Read the model definition and answer for the solid it produces. Units are mm, in the model's axes. Give positions to 0.01 mm unless a question says otherwise; leave off trailing zeros. Write each loop counter-clockwise with the first axis right and the second up, starting at its lowest first coordinate (ties: lowest second). Pieces come first, ordered by that corner, then holes. Notation, with made-up numbers: (60.5, -13.5) -> (102.5, -13.5) arc R12 cw to (102.5, -7.5) -> close; hole circle Ø5 at (-16.75, 33). An arc over 180 degrees is marked (long way). Use a Markdown table: item, result.
from build123d import *

# Parameters (mm, degrees)
BOSS_EXTRUDE1_DEPTH = 2
FILLET1_R           = 3


with BuildPart() as part:
    # Sketch1 → Boss-Extrude1 (new body)
    with BuildSketch(Plane(origin=(0, 0, 0), x_dir=(1, 0, 0), z_dir=(0, 1, 0))):
        Polygon((-160, -197.649746193), (-160, -185.649746193), (0, -185.649746193), (0, -197.649746193), (30, -197.649746193), (30, 34.350253807), (-190, 34.350253807), (-190, -197.649746193), align=None)
    extrude(amount=BOSS_EXTRUDE1_DEPTH)

    # Fillet1
    fillet1_edges = [part.edges().sort_by_distance(p)[0] for p in [
        (-190, 1, -34.350253807),
        (30, 1, -34.350253807),
        (30, 1, 197.649746193),
        (0, 1, 197.649746193),
        (-160, 1, 197.649746193),
        (-190, 1, 197.649746193),
    ]]
    fillet(fillet1_edges, radius=FILLET1_R)


solid = part.part
Item 1: A cutting plane is placed at B-B (x = -27). Give the vertices of the cut face in (y, z).
Return value:
| item | result |
|---|---|
| outline | (0, -34.35) -> (2, -34.35) -> (2, 185.65) -> (0, 185.65) -> close |
Item 2: This flat-tipped pin is pushed along its axis until it touches: P1, Ø1, axis at x = -88.5, y = 1, coming from the +Z side. Where does it stop, or does it pass through?
Return value:
| item | result |
|---|---|
| P1 | z = 185.65 |
Item 3: A straight line is drawn through the part: line 1 along Z through (x, y) = (-1.5, 1.6). Find the intervals that lie inside material, in ascending order. Write a range as [from, to].
Return value:
| item | result |
|---|---|
| line 1 | [-34.35, 185.65] |
Item 4: A cutting plane is placed at A-A (y = 1). Give the vertices of the cut face in (x, z).
Return value:
| item | result |
|---|---|
| outline | (-190, -31.35) arc R3 ccw to (-187, -34.35) -> (27, -34.35) arc R3 ccw to (30, -31.35) -> (30, 194.65) arc R3 ccw to (27, 197.65) -> (3, 197.65) arc R3 ccw to (0, 194.65) -> (0, 185.65) -> (-160, 185.65) -> (-160, 194.65) arc R3 ccw to (-163, 197.65) -> (-187, 197.65) arc R3 ccw to (-190, 194.65) -> close |
Item 5: For a pull along Y with two mould halves and no side action, classify faces 1 (the face through (-82, 2, 80)), 2 (the face through (-82, 0, 80)) as +Y half, -Y half, draft (parallel to the pull), parting line (faces both ways), or undercut.
Return value:
| item | result |
|---|---|
| face 1 | +Y half |
| face 2 | -Y half |
